from build123d import *

# Parameters (mm, degrees)
SKETCH1_W           = 4.2
SKETCH1_H           = 19.5
BOSS_EXTRUDE1_DEPTH = 1.5875


with BuildPart() as part:
    # Sketch1 → Boss-Extrude1 (new body)
    with BuildSketch(Plane(origin=(0, 0, 0), x_dir=(1, 0, 0), z_dir=(0, 1, 0))):
        with BuildLine():
            Line((-27.1, 9.75), (-70, 9.75))
            Line((-70, 9.75), (-70, -9.75))
            Line((-70, -9.75), (-27.1, -9.75))
            Line((-27.1, -9.75), (-27.1, -13.75))
            Line((-27.1, -13.75), (-16.9, -13.75))
            Line((-16.9, -13.75), (-16.9, -9.75))
            Line((-16.9, -9.75), (70, -9.75))
            Line((70, -9.75), (70, 9.75))
            Line((70, 9.75), (47.791477279, 9.75))
            ThreePointArc((47.791477279, 9.75), (28.607181878, 4.414037573), (9.422886477, 9.75))
            Line((9.422886477, 9.75), (-16.9, 9.75))
            Line((-16.9, 9.75), (-16.9, 13.75))
            Line((-16.9, 13.75), (-27.1, 13.75))
            Line((-27.1, 13.75), (-27.1, 9.75))
        make_face()
        with Locations((-22, 0)):
            Rectangle(SKETCH1_W, SKETCH1_H, mode=Mode.SUBTRACT)
    extrude(amount=BOSS_EXTRUDE1_DEPTH)


solid = part.part
Can you work these out from the model? Positions are in its coordinate system, mm. Round coordinates to 2 decimals unless told otherwise and drop trailing zeros. Write each loop counter-clockwise with the first axis right and the second up, starting at its lowest first coordinate (ties: lowest second). Pieces come first, ordered by that corner, then holes. Notation, with made-up numbers: M 5.5,53.25 L 56.5,53.25 A25 ccw 56.5,92.25 Z; hole C 0.25,-38 d6. An arc over 180 degrees is marked long. Use a Markdown table: item, result.
Item 1: For pin 1 Ø0.8 at (y, z) = (1, -11) entering from -X; pin 2 Ø0.5 at (x, y) = (35.5, 1) entering from +Z; pin 3 Ø0.5 at (y, z) = (1, -11.5) entering from +X, each with a flat end and sliding along its axis, tell me the tip position at first contact or that it passes through.
Found:
| item | result |
|---|---|
| pin 1 | stops at x = -27.1 |
| pin 2 | stops at z = 9.75 |
| pin 3 | stops at x = -16.9 |
Item 2: I want a section at C-C (x = 8). List the corners of the cut face in (y, z) for me, and give its area (3 significant figures).
Found:
| item | result |
|---|---|
| outline | M 0,-9.75 L 1.59,-9.75 L 1.59,9.75 L 0,9.75 Z |
| area | 31.0 mm2 |
Item 3: I want a section at D-D (z = -11.75). List the corners of the cut face in (x, y) for me, and give its area (3 significant figures).
Found:
| item | result |
|---|---|
| outline | M -27.1,0 L -16.9,0 L -16.9,1.59 L -27.1,1.59 Z |
| area | 16.2 mm2 |
Item 4: I want a section at B-B (y = 1.25). List the corners of the cut face in (x, z) for me, and give its area (3 significant figures).
Found:
| item | result |
|---|---|
| outline | M -70,-9.75 L -27.1,-9.75 L -27.1,-13.75 L -16.9,-13.75 L -16.9,-9.75 L 9.42,-9.75 A37.15 cw 47.79,-9.75 L 70,-9.75 L 70,9.75 L -16.9,9.75 L -16.9,13.75 L -27.1,13.75 L -27.1,9.75 L -70,9.75 Z; hole M -24.1,-9.75 L -19.9,-9.75 L -19.9,9.75 L -24.1,9.75 Z |
| area | 2,590 mm2 |
Item 5: If I drill on line 1 along X through (y, z) = (0.4, 5); line 2 along X through (y, z) = (0.1, -7.25); line 3 along X through (y, z) = (0.4, -7), over which ranges is the centre line in solid material (lowest first)? Write a range as [from, to].
Found:
| item | result |
|---|---|
| line 1 | x = [-70, -24.1], [-19.9, 70] |
| line 2 | x = [-70, -24.1], [-19.9, 14.37], [42.84, 70] |
| line 3 | x = [-70, -24.1], [-19.9, 14.99], [42.23, 70] |
Item 6: I want a section at A-A (z = 4.75). List the corners of the cut face in (x, y) for me.
Found:
| item | result |
|---|---|
| outline | M -70,0 L -24.1,0 L -24.1,1.59 L -70,1.59 Z; M -19.9,0 L 70,0 L 70,1.59 L -19.9,1.59 Z |
